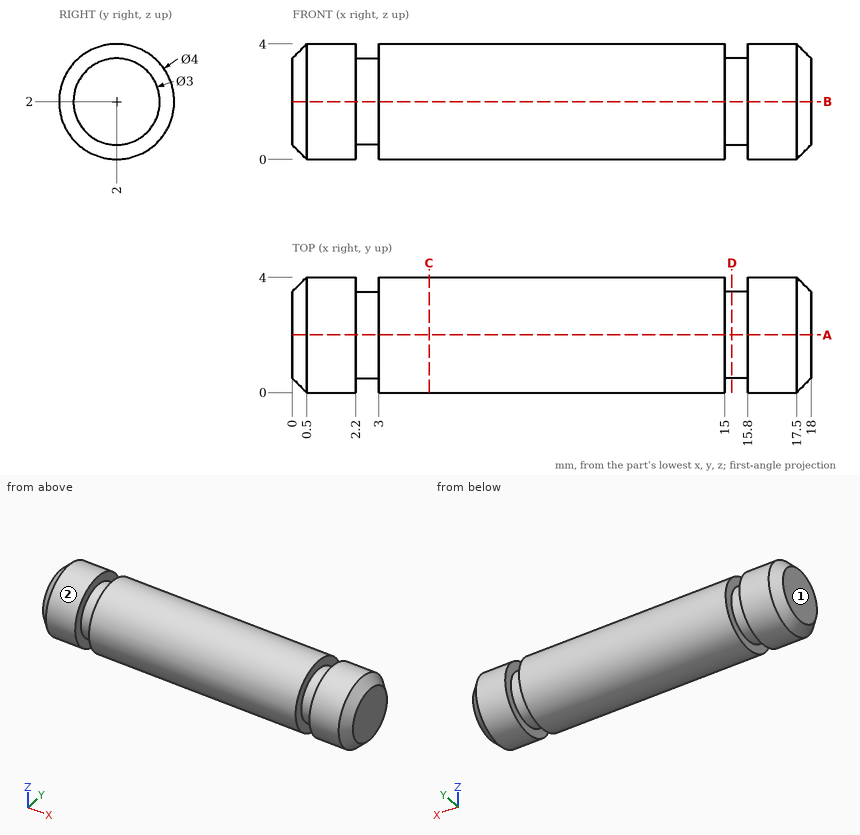
Study the drawing (mm; zero at the part's minimum x, y, z) and answer. Coordinates: 2 decimals unless noted, no trailing zeros. Write each loop counter-clockwise with the first axis right and the second up, starting at its lowest first coordinate (ties: lowest second). Pieces come first, ordered by that corner, then holes. Notation, with made-up numbers: (-19, 50.5) - (36, 50.5) arc R17 cw to (36, 62.5) - close; hole circle Ø6 at (12.25, 38). An arc over 180 degrees is marked (long way). Answer as a JSON object with one key per item and string values. Group by question number.
1. A cutting plane is placed at D-D (x = 15.25). Determine the outline of the cut face in (y, z).
2. A cutting plane is placed at A-A (y = 2). Determine the outline of the cut face in (x, z).
3. Consider L1, parallel to X at y = 2.5, z = 0.35; L2, parallel to X at y = 2.3, z = 3.75; L3, parallel to Y at x = 13.25, z = 1.6. Determine where each line is inside the solid, lowest interval first. Write a range as [from, to].
4. Each of these flat-tipped pins is pushed along its axis until it touches: P1, Ø2, axis at x = 14.5, y = 3.5, coming from the -Z side; P2, Ø1, axis at x = 2.5, z = 3.5, coming from the -Y side; P3, Ø1, axis at x = 2.5, z = 3.5, coming from the +Y side. Where does it stop, or does it pass through?
5. A cutting plane is placed at C-C (x = 4.75). Determine the outline of the cut face in (y, z), plus the area to 3 significant figures.
6. The mould has two halves that part along Z. Classify the marked faces 1 and 2: +Z half, -Z half, draft (parallel to the pull), parting line (faces both ways), or undercut.
Worked out:
{
 "1": {"outline": "circle Ø3 at (2, 2)"},
 "2": {"outline": "(0, 0.5) - (0.5, 0) - (2.2, 0) - (2.2, 0.5) - (3, 0.5) - (3, 0) - (15, 0) - (15, 0.5) - (15.8, 0.5) - (15.8, 0) - (17.5, 0) - (18, 0.5) - (18, 3.5) - (17.5, 4) - (15.8, 4) - (15.8, 3.5) - (15, 3.5) - (15, 4) - (3, 4) - (3, 3.5) - (2.2, 3.5) - (2.2, 4) - (0.5, 4) - (0, 3.5) - close"},
 "3": {"L1": "x = [0.22, 2.2], [3, 15], [15.8, 17.78]", "L2": "x = [0.28, 2.2], [3, 15], [15.8, 17.72]", "L3": "y = [0.04, 3.96]"},
 "4": {"P1": "stops at z = 0.06", "P2": "stops at y = 0.33", "P3": "stops at y = 3.67"},
 "5": {"outline": "circle Ø4 at (2, 2)", "area": "12.6 mm²"},
 "6": {"face 1": "draft", "face 2": "parting line"}
}
